from build123d import *

# Parameters (mm, degrees)
F0_W     = 20
F0_H     = 60
F1_DEPTH = 30
F0_R     = 10
F2_DEPTH = 10
F3_R     = 10
F4_DEPTH = 10


with BuildPart() as f1:
    # F0 (on Front) → F1 (new body, symmetric)
    with BuildSketch(Plane.XZ):
        with Locations((10, 0)):
            Rectangle(F0_W, F0_H)
    extrude(amount=F1_DEPTH, both=True)

    # F0 (on Front) → F2 (join, symmetric)
    with BuildSketch(Plane.XZ):
        with BuildLine():
            Line((0, -30), (0, 30))
            Line((0, 30), (-30, 30))
            ThreePointArc((-30, 30), (-60, 0), (-30, -30))
            Line((-30, -30), (0, -30))
        make_face()
        with Locations((-30, 0)):
            Circle(F0_R, mode=Mode.SUBTRACT)
    extrude(amount=F2_DEPTH, both=True)

    # F3 (on Top) → F4 (join, symmetric)
    with BuildSketch(Plane.XY):
        with BuildLine():
            Line((20, 30), (20, -30))
            Line((20, -30), (50, -30))
            ThreePointArc((50, -30), (80, 0), (50, 30))
            Line((50, 30), (20, 30))
        make_face()
        with Locations((50, 0)):
            Circle(F3_R, mode=Mode.SUBTRACT)
    extrude(amount=F4_DEPTH, both=True)


solid = f1.part
Design review of the part built by this model. Coordinates are the model's own, in mm. A direction names the side the tool comes from. Coordinates: 2 decimals unless noted, no trailing zeros. Order: outer loops, then holes, each group sorted by start corner. A loop starts at its lowest first (then second) coordinate and runs counter-clockwise, first axis right, second up. Notation, with made-up numbers: (8, 14) -> (55, 14) arc R21 ccw to (55, 31) -> close; hole circle Ø8 at (27.5, -32). An arc over 180 degrees is marked (long way). One line per item, written item: value.
1) We need section C-C, the plane x = -26.5. Give the boundary of the cut face in (y, z), then the cut area to 3 significant figures.
Output values:
outline: (-10, -30) -> (10, -30) -> (10, -9.37) -> (-10, -9.37) -> close; (-10, 9.37) -> (10, 9.37) -> (10, 30) -> (-10, 30) -> close
area: 825 mm2
2) Machinability: for faces 4 (the face through (0, 0, 30)), 5 (the face through (36, 0, 10)), 6 (the face through (36, 0, -10)), 7 (the face through (0, 20, 0)), 8 (the face through (0, -20, 0)), which of the approach directions +Z, -Z, +X, -X, +Y, -Y give a long, thin tool a straight path to every point of the face, cutting with its end or side? Answer none if there is none.
Output values:
face 4: +Z, +X, -X, +Y, -Y
face 5: +Z, +X, +Y, -Y
face 6: -Z, +X, +Y, -Y
face 7: +Z, -Z, -X, +Y
face 8: +Z, -Z, -X, -Y
3) We need section D-D, the plane z = -20. Give the boundary of the cut face in (x, y).
Output values:
outline: (-52.36, -10) -> (0, -10) -> (0, -30) -> (20, -30) -> (20, 30) -> (0, 30) -> (0, 10) -> (-52.36, 10) -> close
4) Clearance check with flat-ended pins moving along their axes: P1, Ø18, axis at x = 55, y = 12, coming from the +Z side; P2, Ø10, axis at y = 25, z = -14.5, coming from the -X side; P3, Ø2, axis at x = 36, y = 23.5, coming from the -Z side. State where each tip first meets the part, or that it passes through.
Output values:
P1: stops at z = 10
P2: stops at x = 0
P3: stops at z = -10
5) We need section A-A, the plane y = 0. Give the boundary of the cut face in (x, z), then the cut area to 3 significant figures.
Output values:
outline: (-30, -30) -> (20, -30) -> (20, -10) -> (40, -10) -> (40, 10) -> (20, 10) -> (20, 30) -> (-30, 30) arc R30 ccw to start; (60, -10) -> (80, -10) -> (80, 10) -> (60, 10) -> close; hole circle Ø20 at (-30, 0)
area: 4,900 mm2
6) Draft analysis for pull direction Z (two halves, no side actions). For faces 1 (the face through (0, 0, -30)), 2 (the face through (40, 0, 0)), 3 (the face through (-40, 0, 0)), state which applies: +Z half, -Z half, draft (parallel to the pull), parting line (faces both ways), or undercut.
Output values:
face 1: -Z half
face 2: draft
face 3: undercut
7) To check wall thickness, follow probe 1 along Y at (x, z) = (50, 1); probe 2 along X at (y, z) = (-15, 22.5). State the ranges of each line that lie inside material, in increasing order. Write a range as [from, to].
Output values:
probe 1: y = [-30, -10], [10, 30]
probe 2: x = [0, 20]
8) We need section B-B, the plane z = -6.5. Give the boundary of the cut face in (x, y), then the cut area to 3 significant figures.
Output values:
outline: (-59.29, -10) -> (-37.6, -10) -> (-37.6, 10) -> (-59.29, 10) -> close; (-22.4, -10) -> (0, -10) -> (0, -30) -> (50, -30) arc R30 ccw to (50, 30) -> (0, 30) -> (0, 10) -> (-22.4, 10) -> close; hole circle Ø20 at (50, 0)
area: 4,980 mm2
